For this review, take the finished solid that the model builds, in its own axes (mm). A direction names the side the tool comes from. Round coordinates to 2 decimals unless told otherwise and drop trailing zeros. Loops run counter-clockwise (first coordinate to the right, second up) from the corner with the lowest first, then second, coordinate; pieces in that order, holes last. Notation, with made-up numbers: (-3.75, -18.75) -> (55.25, -18.75) arc R31 cw to (55.25, 10.25) -> close; hole circle Ø6 at (63, -20.75). An arc over 180 degrees is marked (long way). One line per question, with ' | ' between items. Start each with the question number.
1. Draft analysis for pull direction Y (two halves, no side actions). For faces 1 (the face through (21, -27, 3)), 2 (the face through (0, 22, -5.5)), 3 (the face through (-0.238, 11.074, -2.788)), state which applies: pulls with the +Y half, pulls with the -Y half, needs draft (parallel to the pull), parting line crosses it, or undercut.
2. Consider section C-C (z = 5). Count the separate pieces of the cut face and the enclosed holes in it, and give its area (3 significant figures).
3. For faces 4 (the face through (-21.3, -27.3, 7)), 5 (the face through (10.5, 0, -1)), 6 (the face through (9, -20, -1)), list the 3-axis set-ups (+Z, -Z, +X, -X, +Y, -Y) from which the entire face can be reached by the end or side of a thin tool; tool diameter is ignored.
4. For pin 1 Ø8 at (x, z) = (13, 2) entering from +Y; pin 2 Ø1.9 at (x, y) = (11, -21.5) entering from -Z; pin 3 Ø6 at (y, z) = (36.5, 4.5) entering from +X, all flat-tipped, find the tip position at first contact; note any pin that passes through.
5. Consider section B-B (x = 13). Write out the cut boundary in (y, z), and give its area (3 significant figures).
6. Wall thickness on line 1 along X through (y, z) = (-26, 4.25); line 2 along Y through (x, z) = (-4, 11.75); line 3 along Y through (x, z) = (7.9, 5): over which ranges is each line inside the solid? List them lowest first.
7. Consider section A-A (y = 0). Write out the cut boundary in (x, z), and give its area (3 significant figures).
8. Consider section D-D (y = 10). Write out the cut boundary in (x, z).
Autodesk Fusion 360 part; units mm, degrees
ref_plane "工作平面1" through (0, 0, 0) normal (0, 0, 1) x (1, 0, 0)
sketch "草图1" plane through (0, 0, 0) normal (0, 0, 1) x (1, 0, 0)
  line L0 (-26, -22) -> (26, -22)
  line L1 (26, -22) -> (28, -20)
  line L2 (28, -20) -> (28, 20)
  line L3 (28, 20) -> (26, 22)
  line L4 (26, 22) -> (-26, 22)
  line L5 (-26, 22) -> (-28, 20)
  line L6 (-28, 20) -> (-28, -20)
  line L7 (-28, -20) -> (-26, -22)
extrude "56 x 44 x 7 platform" add sketch "草图1" along normal blind 7
ref_plane "工作平面2" through (0, 0, 7) normal (0, 0, 1) x (1, 0, 0)
sketch "草图2" plane through (0, 0, 7) normal (0, 0, 1) x (1, 0, 0)
  line L0 (-28, -22) -> (-20.49, -22)
  line L1 (-20.49, -22) -> (-20.49, 22)
  line L2 (-20.49, 22) -> (-28, 22)
  line L3 (-28, 22) -> (-28, -22)
ref_plane "工作平面3" through (0, 0, 12.2) normal (0, 0, 1) x (1, 0, 0)
sketch "草图3" plane through (0, 0, 12.2) normal (0, 0, 1) x (1, 0, 0)
  line L0 (-28, -22) -> (-16.33, -22)
  line L1 (-16.33, -22) -> (-16.33, 22)
  line L2 (-16.33, 22) -> (-28, 22)
  line L3 (-28, 22) -> (-28, -22)
loft "Dovetail retaining rail 0.8 to 1 -1" add profiles "草图2", "草图3" section 1 section 2
ref_plane "工作平面4" through (0, 0, 6.7) normal (0, 0, 1) x (1, 0, 0)
sketch "草图4" plane through (0, 0, 6.7) normal (0, 0, 1) x (1, 0, 0)
  line L0 (-23.4, -22) -> (-22.5, -22)
  line L1 (-22.5, -22) -> (-22.5, 13)
  line L2 (-22.5, 13) -> (-23.4, 13)
  line L3 (-23.4, 13) -> (-23.4, -22)
extrude "0.9 mm longitudinal flexure slot -1" cut sketch "草图4" along normal blind 5.8
ref_plane "工作平面5" through (0, 0, 6.7) normal (0, 0, 1) x (1, 0, 0)
sketch "草图5" plane through (0, 0, 6.7) normal (0, 0, 1) x (1, 0, 0)
  line L0 (-22.5, -22) -> (-15, -22)
  line L1 (-15, -22) -> (-15, 13)
  line L2 (-15, 13) -> (-22.5, 13)
  line L3 (-22.5, 13) -> (-22.5, -22)
extrude "0.8 mm flexure underside relief -1" cut sketch "草图5" along normal blind 0.8
ref_plane "工作平面6" through (0, 0, 7.6) normal (0, 0, 1) x (1, 0, 0)
sketch "草图6" plane through (0, 0, 7.6) normal (0, 0, 1) x (1, 0, 0)
  line L0 (-20.21, -6) -> (-20.21, 11)
  line L1 (-20.21, 11) -> (-19.66, 11)
  line L2 (-19.66, 11) -> (-19.66, 2)
  line L3 (-19.66, 2) -> (-20.11, -6)
  line L4 (-20.11, -6) -> (-20.21, -6)
ref_plane "工作平面7" through (0, 0, 11.8) normal (0, 0, 1) x (1, 0, 0)
sketch "草图7" plane through (0, 0, 11.8) normal (0, 0, 1) x (1, 0, 0)
  line L0 (-16.85, -6) -> (-16.85, 11)
  line L1 (-16.85, 11) -> (-16.3, 11)
  line L2 (-16.3, 11) -> (-16.3, 2)
  line L3 (-16.3, 2) -> (-16.75, -6)
  line L4 (-16.75, -6) -> (-16.85, -6)
loft "Tapered friction contact rib -1" add profiles "草图6", "草图7" section 1 section 2
ref_plane "工作平面8" through (0, 0, 7) normal (0, 0, 1) x (1, 0, 0)
sketch "草图8" plane through (0, 0, 7) normal (0, 0, 1) x (1, 0, 0)
  line L0 (20.49, -22) -> (28, -22)
  line L1 (28, -22) -> (28, 22)
  line L2 (28, 22) -> (20.49, 22)
  line L3 (20.49, 22) -> (20.49, -22)
ref_plane "工作平面9" through (0, 0, 12.2) normal (0, 0, 1) x (1, 0, 0)
sketch "草图9" plane through (0, 0, 12.2) normal (0, 0, 1) x (1, 0, 0)
  line L0 (16.33, -22) -> (28, -22)
  line L1 (28, -22) -> (28, 22)
  line L2 (28, 22) -> (16.33, 22)
  line L3 (16.33, 22) -> (16.33, -22)
loft "Dovetail retaining rail 0.8 to 1 1" add profiles "草图8", "草图9" section 1 section 2
ref_plane "工作平面10" through (0, 0, 6.7) normal (0, 0, 1) x (1, 0, 0)
sketch "草图10" plane through (0, 0, 6.7) normal (0, 0, 1) x (1, 0, 0)
  line L0 (22.5, -22) -> (23.4, -22)
  line L1 (23.4, -22) -> (23.4, 13)
  line L2 (23.4, 13) -> (22.5, 13)
  line L3 (22.5, 13) -> (22.5, -22)
extrude "0.9 mm longitudinal flexure slot 1" cut sketch "草图10" along normal blind 5.8
ref_plane "工作平面11" through (0, 0, 6.7) normal (0, 0, 1) x (1, 0, 0)
sketch "草图11" plane through (0, 0, 6.7) normal (0, 0, 1) x (1, 0, 0)
  line L0 (15, -22) -> (22.5, -22)
  line L1 (22.5, -22) -> (22.5, 13)
  line L2 (22.5, 13) -> (15, 13)
  line L3 (15, 13) -> (15, -22)
extrude "0.8 mm flexure underside relief 1" cut sketch "草图11" along normal blind 0.8
ref_plane "工作平面12" through (0, 0, 7.6) normal (0, 0, 1) x (1, 0, 0)
sketch "草图12" plane through (0, 0, 7.6) normal (0, 0, 1) x (1, 0, 0)
  line L0 (20.21, -6) -> (20.21, 11)
  line L1 (20.21, 11) -> (19.66, 11)
  line L2 (19.66, 11) -> (19.66, 2)
  line L3 (19.66, 2) -> (20.11, -6)
  line L4 (20.11, -6) -> (20.21, -6)
ref_plane "工作平面13" through (0, 0, 11.8) normal (0, 0, 1) x (1, 0, 0)
sketch "草图13" plane through (0, 0, 11.8) normal (0, 0, 1) x (1, 0, 0)
  line L0 (16.85, -6) -> (16.85, 11)
  line L1 (16.85, 11) -> (16.3, 11)
  line L2 (16.3, 11) -> (16.3, 2)
  line L3 (16.3, 2) -> (16.75, -6)
  line L4 (16.75, -6) -> (16.85, -6)
loft "Tapered friction contact rib 1" add profiles "草图12", "草图13" section 1 section 2
ref_plane "工作平面14" through (0, 0, 7) normal (0, 0, 1) x (1, 0, 0)
sketch "草图14" plane through (0, 0, 7) normal (0, 0, 1) x (1, 0, 0)
  line L0 (-16.5, 19.4) -> (16.5, 19.4)
  line L1 (16.5, 19.4) -> (16.5, 22)
  line L2 (16.5, 22) -> (-16.5, 22)
  line L3 (-16.5, 22) -> (-16.5, 19.4)
extrude "Closed insertion end stop" add sketch "草图14" along normal blind 5.2
ref_plane "工作平面15" through (0, 0, 0) normal (0, 0, 1) x (1, 0, 0)
sketch "草图15" plane through (0, 0, 0) normal (0, 0, 1) x (1, 0, 0)
  circle A0 centre (0, 0) radius 7.5
extrude "15 mm screw and driver access" cut sketch "草图15" along normal blind 7
move_body "Align camera long edge with gimbal arm - 90 degrees" bodies 1 to x (0, 1, 0) y (-1, 0, 0) z (0, 0, 1) at (0, 0, 0)
ref_plane "工作平面16" through (0, 0, 0) normal (0, 0, 1) x (1, 0, 0)
sketch "草图16" plane through (0, 0, 0) normal (0, 0, 1) x (1, 0, 0)
  line L0 (7.8, -28) -> (11.4, -28)
  line L1 (11.4, -28) -> (11.4, -21.95)
  line L2 (11.4, -21.95) -> (7.8, -21.95)
  line L3 (7.8, -21.95) -> (7.8, -28)
extrude "Clear original raised tab and root fillet" cut sketch "草图16" along normal blind 12.3
ref_plane "工作平面17" through (0, 0, 0) normal (0, 0, 1) x (1, 0, 0)
sketch "草图17" plane through (0, 0, 0) normal (0, 0, 1) x (1, 0, 0)
  line L0 (7.8, 25.95) -> (11.4, 25.95)
  line L1 (11.4, 25.95) -> (11.4, 28)
  line L2 (11.4, 28) -> (7.8, 28)
  line L3 (7.8, 28) -> (7.8, 25.95)
extrude "Clear original raised tab and root fillet (1)" cut sketch "草图17" along normal blind 12.3
ref_plane "工作平面18" through (0, 0, -2.1) normal (0, 0, 1) x (1, 0, 0)
sketch "草图18" plane through (0, 0, -2.1) normal (0, 0, 1) x (1, 0, 0)
  line L0 (-8.5, -20) -> (-6.3, -20)
  line L1 (-6.3, -20) -> (-6.3, 20)
  line L2 (-6.3, 20) -> (-8.5, 20)
  line L3 (-8.5, 20) -> (-8.5, -20)
extrude "Arm lateral locating shoulder" add sketch "草图18" along normal blind 2.1
ref_plane "工作平面19" through (0, 0, -2.1) normal (0, 0, 1) x (1, 0, 0)
sketch "草图19" plane through (0, 0, -2.1) normal (0, 0, 1) x (1, 0, 0)
  line L0 (8.3, -20) -> (10.5, -20)
  line L1 (10.5, -20) -> (10.5, 20)
  line L2 (10.5, 20) -> (8.3, 20)
  line L3 (8.3, 20) -> (8.3, -20)
extrude "Arm lateral locating shoulder (1)" add sketch "草图19" along normal blind 2.1
ref_plane "工作平面20" through (0, 0, -5.5) normal (0, 0, 1) x (1, 0, 0)
sketch "草图20" plane through (0, 0, -5.5) normal (0, 0, 1) x (1, 0, 0)
  circle A0 centre (0, -22) radius 1.1
extrude "Reinforced 2.2 x 5.5 mm heat stake pin at arm y -22" add sketch "草图20" along normal blind 5.5
ref_plane "工作平面21" through (0, 0, -5.5) normal (0, 0, 1) x (1, 0, 0)
sketch "草图21" plane through (0, 0, -5.5) normal (0, 0, 1) x (1, 0, 0)
  circle A0 centre (0, -10) radius 1.1
extrude "Reinforced 2.2 x 5.5 mm heat stake pin at arm y -10" add sketch "草图21" along normal blind 5.5
ref_plane "工作平面22" through (0, 0, -5.5) normal (0, 0, 1) x (1, 0, 0)
sketch "草图22" plane through (0, 0, -5.5) normal (0, 0, 1) x (1, 0, 0)
  circle A0 centre (0, 10) radius 1.1
extrude "Reinforced 2.2 x 5.5 mm heat stake pin at arm y 10" add sketch "草图22" along normal blind 5.5
ref_plane "工作平面23" through (0, 0, -5.5) normal (0, 0, 1) x (1, 0, 0)
sketch "草图23" plane through (0, 0, -5.5) normal (0, 0, 1) x (1, 0, 0)
  circle A0 centre (0, 22) radius 1.1
extrude "Reinforced 2.2 x 5.5 mm heat stake pin at arm y 22" add sketch "草图23" along normal blind 5.5
ref_plane "工作平面24" through (0, 0, 0) normal (0, 0, 1) x (1, 0, 0)
sketch "草图24" plane through (0, 0, 0) normal (0, 0, 1) x (1, 0, 0)
  line L0 (5, -32.15) -> (8.7, -32.15)
  line L1 (8.7, -32.15) -> (8.7, -24.15)
  line L2 (8.7, -24.15) -> (5, -24.15)
  line L3 (5, -24.15) -> (5, -32.15)
extrude "Ear for original 3.2 mm side hole at arm y -28.15" add sketch "草图24" along normal blind 7.2
ref_plane "工作平面25" through (0, 0, 0) normal (0, 0, 1) x (1, 0, 0)
sketch "草图25" plane through (0, 0, 0) normal (0, 0, 1) x (1, 0, 0)
  line L0 (7.8, -32.15) -> (8.9, -32.15)
  line L1 (8.9, -32.15) -> (8.9, -24.15)
  line L2 (8.9, -24.15) -> (7.8, -24.15)
  line L3 (7.8, -24.15) -> (7.8, -32.15)
extrude "Ear relief around original arm root radius" cut sketch "草图25" along normal blind 1.3
ref_plane "工作平面26" through (4.9, 0, 0) normal (1, 0, 0) x (0, 1, 0)
sketch "草图26" plane through (4.9, 0, 0) normal (1, 0, 0) x (0, 0, -1)
  circle A0 centre (-5, -28.15) radius 1.6
extrude "Side rivet ear clearance" cut sketch "草图26" along normal blind 4
ref_plane "工作平面27" through (0, 0, 0) normal (0, 0, 1) x (1, 0, 0)
sketch "草图27" plane through (0, 0, 0) normal (0, 0, 1) x (1, 0, 0)
  line L0 (5, 27.5) -> (8.7, 27.5)
  line L1 (8.7, 27.5) -> (8.7, 40.85)
  line L2 (8.7, 40.85) -> (5, 40.85)
  line L3 (5, 40.85) -> (5, 27.5)
extrude "Ear for original 3.2 mm side hole at arm y 36.85" add sketch "草图27" along normal blind 7.2
ref_plane "工作平面28" through (0, 0, 0) normal (0, 0, 1) x (1, 0, 0)
sketch "草图28" plane through (0, 0, 0) normal (0, 0, 1) x (1, 0, 0)
  line L0 (7.8, 27.5) -> (8.9, 27.5)
  line L1 (8.9, 27.5) -> (8.9, 40.85)
  line L2 (8.9, 40.85) -> (7.8, 40.85)
  line L3 (7.8, 40.85) -> (7.8, 27.5)
extrude "Ear relief around original arm root radius (1)" cut sketch "草图28" along normal blind 1.3
ref_plane "工作平面29" through (4.9, 0, 0) normal (1, 0, 0) x (0, 1, 0)
sketch "草图29" plane through (4.9, 0, 0) normal (1, 0, 0) x (0, 0, -1)
  circle A0 centre (-5, 36.85) radius 1.6
extrude "Side rivet ear clearance (1)" cut sketch "草图29" along normal blind 4
ref_plane "工作平面30" through (4.9, 0, 0) normal (1, 0, 0) x (0, 1, 0)
sketch "草图30" plane through (4.9, 0, 0) normal (1, 0, 0) x (0, 0, -1)
  circle A0 centre (-5, -28.15) radius 1.6
extrude "Side rivet full passage clearance" cut sketch "草图30" along normal blind 20
ref_plane "工作平面31" through (2.9, 0, 0) normal (1, 0, 0) x (0, 1, 0)
sketch "草图31" plane through (2.9, 0, 0) normal (1, 0, 0) x (0, 0, -1)
  circle A0 centre (-5, -28.15) radius 2.9
extrude "Side rivet flange counterbore" cut sketch "草图31" along normal blind 2.2
ref_plane "工作平面32" through (4.9, 0, 0) normal (1, 0, 0) x (0, 1, 0)
sketch "草图32" plane through (4.9, 0, 0) normal (1, 0, 0) x (0, 0, -1)
  circle A0 centre (-5, 36.85) radius 1.6
ref_plane "工作平面33" through (2.9, 0, 0) normal (1, 0, 0) x (0, 1, 0)
sketch "草图33" plane through (2.9, 0, 0) normal (1, 0, 0) x (0, 0, -1)
  circle A0 centre (-5, 36.85) radius 2.9
extrude "Side rivet flange counterbore (1)" cut sketch "草图33" along normal blind 2.2
Answer block:
1) face 1: pulls with the -Y half | face 2: needs draft | face 3: undercut
2) separate pieces: 3 | enclosed holes: 1 | area: 2,270 mm2
3) face 4: -Z, -X, -Y | face 5: -Z, +X, +Y, -Y | face 6: -Z, +X, -X, -Y
4) pin 1: stops at y = 28 | pin 2: stops at z = 0 | pin 3: stops at x = 8.7
5) outline: (-28, 0) -> (28, 0) -> (28, 12.2) -> (23.4, 12.2) -> (23.4, 6.7) -> (15, 6.7) -> (15, 7) -> (-15, 7) -> (-15, 6.7) -> (-23.4, 6.7) -> (-23.4, 12.2) -> (-28, 12.2) -> (-28, 6.59) arc R1.6 cw to (-28, 3.41) -> close; (-22.5, 7.5) -> (-20.09, 7.5) -> (-16.33, 12.2) -> (-22.5, 12.2) -> close; (16.33, 12.2) -> (20.09, 7.5) -> (22.5, 7.5) -> (22.5, 12.2) -> close | area: 472 mm2
6) line 1: x = -22 to 2.9, 5.1 to 8.7, 11.4 to 22 | line 2: y = -28 to -23.4, -22.5 to -16.34, 16.34 to 22.5, 23.4 to 28 | line 3: y = -32.15 to -29.75, -26.55 to -24.15, -21.95 to 25.95, 27.5 to 35.25, 38.45 to 40.85
7) outline: (-22, 0) -> (-8.5, 0) -> (-8.5, -2.1) -> (-6.3, -2.1) -> (-6.3, 0) -> (-7.5, 0) -> (-7.5, 7) -> (-19.4, 7) -> (-19.4, 12.2) -> (-22, 12.2) -> close; (7.5, 0) -> (8.3, 0) -> (8.3, -2.1) -> (10.5, -2.1) -> (10.5, 0) -> (22, 0) -> (22, 7) -> (7.5, 7) -> close | area: 226 mm2
8) outline: (-22, 0) -> (-8.5, 0) -> (-8.5, -2.1) -> (-6.3, -2.1) -> (-6.3, 0) -> (-1.1, 0) -> (-1.1, -5.5) -> (1.1, -5.5) -> (1.1, 0) -> (8.3, 0) -> (8.3, -2.1) -> (10.5, -2.1) -> (10.5, 0) -> (22, 0) -> (22, 7) -> (-19.4, 7) -> (-19.4, 12.2) -> (-22, 12.2) -> close
